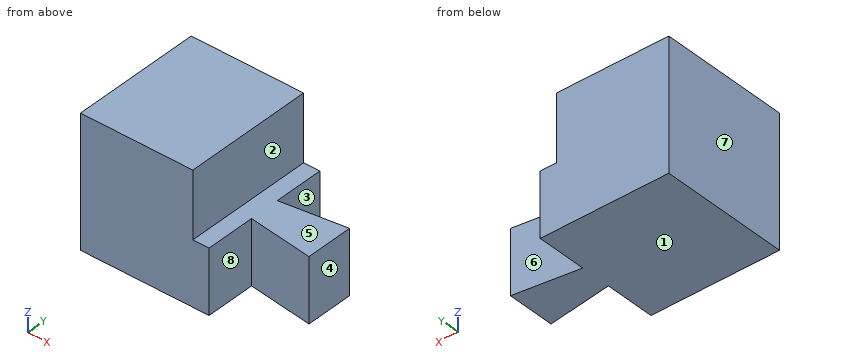
Autodesk Inventor part; units mm, degrees
ref_plane "YZ Plane" through (0, 0, 0) normal (1, 0, 0) x (0, 1, 0)
ref_plane "XZ Plane" through (0, 0, 0) normal (0, 1, 0) x (-1, 0, 0)
ref_plane "XY Plane" through (0, 0, 0) normal (0, 0, 1) x (1, 0, 0)
sketch "Boceto1" plane through (0, 0, 0) normal (0, 0, 1) x (1, 0, 0)
  line L0 (0, 0) -> (0, 40)
  line L1 (0, 40) -> (39.65, 40)
  line L2 (0, 0) -> (39.65, 0)
  line L3 (39.65, 0) -> (39.65, 15.35)
  line L4 (39.65, 40) -> (39.65, 24.65)
  line L5 (39.65, 0) -> (59.65, 0) construction
  line L6 (39.65, 40) -> (59.65, 40) construction
  line L7 (59.65, 40) -> (59.65, 27.325) construction
  line L8 (59.65, 0) -> (59.65, 12.675) construction
  line L9 (39.65, 24.65) -> (59.65, 27.325)
  line L10 (39.65, 15.35) -> (59.65, 12.675)
  line L11 (59.65, 12.675) -> (59.65, 27.325)
  dimension "d0" = 40
  dimension "d1" = 39.65
  dimension "d2" = 39.65
  dimension "d3" = 15.35
  dimension "d4" = 15.35
  dimension "d5" = 20
  dimension "d6" = 20
  dimension "d7" = 12.675
  dimension "d8" = 12.675
extrude "Extrusión1" add sketch "Boceto1" along normal blind 40
sketch "Boceto2" plane through (0, 0, 40) normal (0, 0, 1) x (1, 0, 0)
  line L0 (0, 0) -> (34.65, 0)
  line L1 (0, 0) -> (39.65, 0)
  line L2 (34.65, 0) -> (59.65, 0)
  line L3 (59.65, 0) -> (59.65, 40)
  line L4 (59.65, 40) -> (34.65, 40)
  line L5 (39.65, 40) -> (0, 40)
  line L6 (34.65, 0) -> (34.65, 40)
  dimension "d11" = 34.65
  dimension "d12" = 25
  dimension "d13" = 40
  dimension "d14" = 25
extrude "Extrusión2" cut sketch "Boceto2" against normal blind 20.35
equation "\"d12\" = Ancho_corte"
equation "\"d14\" = Ancho_corte"
equation "\"Largo_corte\" = 35"
equation "\"Ancho_corte\" = 25"
equation "\"Angulo_0\" = 0"
properties part number "Macho_parametrizado"
The model under review builds one solid part; all positions refer to its coordinate system, in mm. Face numbers are marked on the shaded views. A direction names the side the tool comes from. Give positions to 0.01 mm unless a question says otherwise; leave off trailing zeros. Write each loop counter-clockwise with the first axis right and the second up, starting at its lowest first coordinate (ties: lowest second). Pieces come first, ordered by that corner, then holes.
(1) Tool access review of the marked faces 4, 5, 6, 7 and 8: name each direction out of +Z, -Z, +X, -X, +Y, -Y from which nothing blocks a thin tool from reaching the whole face with its end or side.
(2) For P1, Ø8, axis at x = 25.5, z = 9, coming from the -Y side; P2, Ø7.5, axis at y = 4, z = 7.5, coming from the +X side; P3, Ø12.5, axis at x = 50, y = 18.5, coming from the +Z side; P4, Ø4, axis at x = 43, z = 8, coming from the -Y side, all flat-tipped, find the tip position at first contact; note any pin that passes through.
(3) To check wall thickness, follow L1, parallel to X at y = 34, z = 17; L2, parallel to X at y = 3, z = 20; L3, parallel to Z at x = 57, y = 19. State the ranges of each line that lie inside material, in increasing order.
(4) Consider section A-A, the plane z = 18. Give the boundary of the cut face in (x, y) (3 decimals), and give its area (3 significant figures).
(5) The part is to be moulded in two halves that separate along X. For the marked faces 1, 2 and 3, say which applies: released by +X, released by -X, zero draft, split by the parting line, or undercut.
(6) Consider section B-B, the plane y = 30. Give the boundary of the cut face in (x, z), and give its area (3 significant figures).
(7) Consider section C-C, the plane x = 42.5. Give the boundary of the cut face in (y, z).
(8) Consider section D-D, the plane z = 36.5. Give the boundary of the cut face in (x, y).
Returned:
1. face 4: +Z, -Z, +X, +Y, -Y
1. face 5: +Z, +X, +Y, -Y
1. face 6: +Z, -Z, +Y
1. face 7: +Z, -Z, -X, +Y, -Y
1. face 8: +Z, -Z, -Y
2. P1: stops at y = 0
2. P2: stops at x = 39.65
2. P3: stops at z = 19.65
2. P4: stops at y = 14.63
3. L1: x = 0 to 39.65
3. L2: x = 0 to 34.65
3. L3: z = 0 to 19.65
4. outline: (0, 0) - (39.65, 0) - (39.65, 15.35) - (59.65, 12.675) - (59.65, 27.325) - (39.65, 24.65) - (39.65, 40) - (0, 40) - close
4. area: 1,830 mm2
5. face 1: zero draft
5. face 2: released by +X
5. face 3: undercut
6. outline: (0, 0) - (39.65, 0) - (39.65, 19.65) - (34.65, 19.65) - (34.65, 40) - (0, 40) - close
6. area: 1,480 mm2
7. outline: (14.97, 0) - (25.03, 0) - (25.03, 19.65) - (14.97, 19.65) - close
8. outline: (0, 0) - (34.65, 0) - (34.65, 40) - (0, 40) - close
